```python
from build123d import *

# Parameters (mm, degrees)
SKETCH_3_R           = 40
EXTRUDE_1_DEPTH      = 4
SKETCH_4_R           = 42.5
EXTRUDE_2_DEPTH      = 1
EXTRUDE_3_DEPTH      = 2
EXTRUDE_3_DEPTH_BACK = 2
SKETCH_5_R           = 2.5


with BuildPart() as part:
    # Sketch 3 → Extrude 1 (new body)
    with BuildSketch(Plane(origin=(0, 0, 0), x_dir=(1, 0, 0), z_dir=(0, 1, 0))):
        with Locations(Location((0, 0, 0), (0, 0, 270))):
            Circle(SKETCH_3_R)
    extrude(amount=EXTRUDE_1_DEPTH)

    # Sketch 4 → Extrude 2 (add)
    with BuildSketch(Plane(origin=(0, 4, 0), x_dir=(1, 0, 0), z_dir=(0, 1, 0))):
        with Locations(Location((0, 0, 0), (0, 0, 270))):
            Circle(SKETCH_4_R)
    extrude(amount=EXTRUDE_2_DEPTH)

    # Sketch 5 → Extrude 3 (add, two sides: drawn at the far end of the back side and taken through both)
    with BuildSketch(Plane(origin=(0, 0, 0), x_dir=(0, 0, -1), z_dir=(1, 0, 0)).offset(-EXTRUDE_3_DEPTH_BACK)):
        with BuildLine():
            add(Edge.make_bspline(
                [(-3.5, 8.517823555), (-3.350300092, 5.23093062), (-6.389981791, 5)],
                knots=[0, 0, 0, 0.868708242, 0.868708242, 0.868708242], degree=2))
            Line((-6.389981791, 5), (6.389981791, 5))
            add(Edge.make_bspline(
                [(3.5, 8.517823555), (3.350300092, 5.23093062), (6.389981791, 5)],
                knots=[0, 0, 0, 0.868708242, 0.868708242, 0.868708242], degree=2))
            add(Edge.make_bspline(
                [(3.5, 15.517823555), (1.510674253, 12.017823555), (3.5, 8.517823555)],
                knots=[0, 0, 0, 1, 1, 1], degree=2))
            ThreePointArc((3.5, 15.517823555), (0, 19.017823555), (-3.5, 15.517823555))
            add(Edge.make_bspline(
                [(-3.5, 15.517823555), (-1.510674253, 12.017823555), (-3.5, 8.517823555)],
                knots=[0, 0, 0, 1, 1, 1], degree=2))
        make_face()
        with Locations((0, 8.517823555)):
            Circle(SKETCH_5_R, mode=Mode.SUBTRACT)
        with Locations((0, 15.517823555)):
            Circle(SKETCH_5_R, mode=Mode.SUBTRACT)
    extrude(amount=EXTRUDE_3_DEPTH + EXTRUDE_3_DEPTH_BACK)


solid = part.part
```
Model file for the job. Use its own axes, mm. A direction names the side the tool comes from. Coordinates: 2 decimals unless noted, no trailing zeros. Loops run counter-clockwise (first coordinate to the right, second up) from the corner with the lowest first, then second, coordinate; pieces in that order, holes last. Notation, with made-up numbers: (-9, 59) - (47, 59) arc R16 cw to (47, 70) - close; hole circle Ø2 at (-28.75, 6). An arc over 180 degrees is marked (long way). Answer as a JSON object with one key per item and string values. Group by question number.
(1) Flat gauge pins, fed straight in: pin 1 (10 mm diameter, centred on y = 11.5, z = -2.5, fed in from +X); pin 2 (2 mm diameter, centred on x = -23.5, y = 5, fed in from -Z); pin 3 (4 mm diameter, centred on x = -8, z = 2.5, fed in from +Y); pin 4 (4 mm diameter, centred on y = 8.52, z = 0, fed in from -X). Where does each tip first touch, or does it go through?
(2) Cut at A-A (z = 0). Give the cut face in (x, y).
(3) Probe line 1 along Y through (x, z) = (0, 0); line 2 along X through (y, z) = (12, 1); line 3 along Y through (x, z) = (5.5, 15.5). List the from-to ranges inside material, lowest first.
(4) Cut at B-B (y = 16.5). Give the cut face in (x, z), then the cut area to 3 significant figures.
(5) Cut at C-C (x = -14). Give the cut face in (y, z), then the cut area to 3 significant figures.
(6) Tool access for faces 1 (the face through (2, 11, 1)), 2 (the face through (-0.028, 19.017, -0.077)), 3 (the face through (-2, 11, 1)), 4 (the face through (-25.861, 4.493, -33.727)), 5 (the face through (-28, 4, -29)): list every direction of +Z, -Z, +X, -X, +Y, -Y with a clear straight run to the whole face (end or side of a thin tool).
(7) Cut at D-D (x = 0). State how many separate pieces and enclosed holes the cut face has, then the cut area to 3 significant figures.
Geometry says:
{
 "1": {"pin 1": "stops at x = 2", "pin 2": "stops at z = -36.06", "pin 3": "stops at y = 5", "pin 4": "passes through"},
 "2": {"outline": "(-42.5, 4) - (-40, 4) - (-40, 0) - (40, 0) - (40, 4) - (42.5, 4) - (42.5, 5) - (2, 5) - (2, 6.02) - (-2, 6.02) - (-2, 5) - (-42.5, 5) - close; (-2, 11.02) - (2, 11.02) - (2, 13.02) - (-2, 13.02) - close; (-2, 18.02) - (2, 18.02) - (2, 19.02) - (-2, 19.02) - close"},
 "3": {"line 1": "y = 0 to 6.02, 11.02 to 13.02, 18.02 to 19.02", "line 2": "x = -2 to 2", "line 3": "y = 0 to 5"},
 "4": {"outline": "(-2, -3.36) - (2, -3.36) - (2, -2.3) - (-2, -2.3) - close; (-2, 2.3) - (2, 2.3) - (2, 3.36) - (-2, 3.36) - close", "area": "8.48 mm^2"},
 "5": {"outline": "(0, -37.47) - (4, -37.47) - (4, -40.13) - (5, -40.13) - (5, 40.13) - (4, 40.13) - (4, 37.47) - (0, 37.47) - close", "area": "380 mm^2"},
 "6": {"face 1": "+Z, -Z, +X, +Y", "face 2": "+X, -X, +Y", "face 3": "+Z, -Z, -X, +Y", "face 4": "+Y, -Y", "face 5": "-Y"},
 "7": {"separate pieces": "1", "enclosed holes": "2", "area": "453 mm^2"}
}
